Drawing for the job (mm, zero at the part's lowest x, y, z). A direction names the side the tool comes from. Coordinates: 2 decimals unless noted, no trailing zeros. Write each loop counter-clockwise with the first axis right and the second up, starting at its lowest first coordinate (ties: lowest second). Pieces come first, ordered by that corner, then holes.
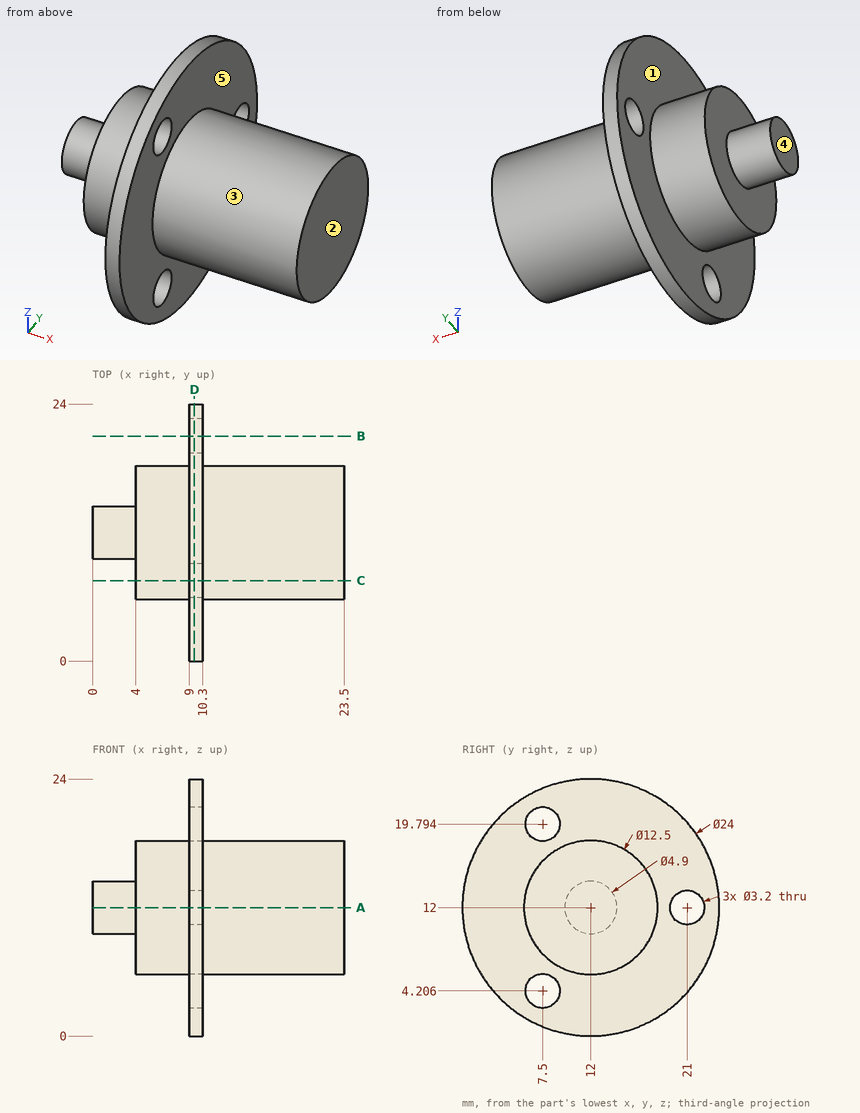
Item 1: Saw through at A-A, the plane z = 12. Write the cut outline in (x, y).
Item 2: Saw through at B-B, the plane y = 21. Write the cut outline in (x, z), and give its area (3 significant figures).
Item 3: Saw through at D-D, the plane x = 9.5. Write the cut outline in (y, z).
Item 4: Wall check: line 1 along Y through (x, z) = (9.45, 12); line 2 along X through (y, z) = (8.5, 8.25); line 3 along X through (y, z) = (11.5, 22.75). Give the ranges that are in metal, low to high.
Item 5: Two-plate mould, pull along X, no slides. Class the marked faces 3, 4 and 5: +X half, -X half, draft (parallel to the pull), parting line (faces both ways), or undercut.
Item 6: Flat gauge pins, fed straight in: pin 1 Ø1.5 at (x, z) = (7.5, 7.5) entering from -Y; pin 2 Ø5 at (y, z) = (21, 12) entering from +X; pin 3 Ø5 at (y, z) = (7.5, 19.79) entering from -X; pin 4 Ø3 at (y, z) = (7.5, 4.21) entering from -X. Where does each tip first touch, or does it go through?
Item 7: Saw through at C-C, the plane y = 7.5. Write the cut outline in (x, z).
Item 8: Which spindle directions (+Z, -Z, +X, -X, +Y, -Y) get a long thin tool onto all of the face, cutting with end or side? Do the marked faces 1 and 2. Say none if no direction does.
Working result:
1. outline: (0, 9.55) - (4, 9.55) - (4, 5.75) - (9, 5.75) - (9, 0) - (10.3, 0) - (10.3, 5.75) - (23.5, 5.75) - (23.5, 18.25) - (10.3, 18.25) - (10.3, 19.4) - (9, 19.4) - (9, 18.25) - (4, 18.25) - (4, 14.45) - (0, 14.45) - close; (9, 22.6) - (10.3, 22.6) - (10.3, 24) - (9, 24) - close
2. outline: (9, 4.06) - (10.3, 4.06) - (10.3, 10.4) - (9, 10.4) - close; (9, 13.6) - (10.3, 13.6) - (10.3, 19.94) - (9, 19.94) - close
2. area: 16.5 mm2
3. outline: circle Ø24 at (12, 12); hole circle Ø3.2 at (7.5, 4.21); hole circle Ø3.2 at (7.5, 19.79); hole circle Ø3.2 at (21, 12)
4. line 1: y = 0 to 19.4, 22.6 to 24
4. line 2: x = 4 to 23.5
4. line 3: x = 9 to 10.3
5. face 3: draft
5. face 4: -X half
5. face 5: +X half
6. pin 1: stops at y = 7
6. pin 2: stops at x = 10.3
6. pin 3: stops at x = 9
6. pin 4: passes through
7. outline: (4, 7.66) - (9, 7.66) - (9, 5.81) - (10.3, 5.81) - (10.3, 7.66) - (23.5, 7.66) - (23.5, 16.34) - (10.3, 16.34) - (10.3, 18.19) - (9, 18.19) - (9, 16.34) - (4, 16.34) - close; (9, 0.88) - (10.3, 0.88) - (10.3, 2.61) - (9, 2.61) - close; (9, 21.39) - (10.3, 21.39) - (10.3, 23.12) - (9, 23.12) - close
8. face 1: -X
8. face 2: +Z, -Z, +X, +Y, -Y
